The listing builds one solid part. Answer for the finished solid, in the listing's coordinates (mm). Give positions to 0.01 mm unless a question says otherwise; leave off trailing zeros. Loops run counter-clockwise (first coordinate to the right, second up) from the corner with the lowest first, then second, coordinate; pieces in that order, holes last. Notation, with made-up numbers: (76.5, -12.5) - (105.5, -12.5) arc R24 ccw to (105.5, 5.5) - close; hole circle Ø10 at (64, 1.25). An arc over 180 degrees is marked (long way). Write each question's results on one line, items separated by ' | '.
from build123d import *

# Parameters (mm, degrees)
F0_W     = 45
F0_H     = 60
F1_DEPTH = 3


with BuildPart() as f1:
    # F0 (on Top) → F1 (new body)
    with BuildSketch(Plane.XY):
        Rectangle(F0_W, F0_H)
        with BuildLine():
            ThreePointArc((-13.6944653346, -25.298272824), (-15.6944653346, -27.298272824), (-17.6944653346, -25.298272824))
            Line((-17.6944653346, -25.298272824), (-17.6944653346, -21.298272824))
            ThreePointArc((-17.6944653346, -21.298272824), (-17.1086788969, -19.8840592617), (-15.6944653346, -19.298272824))
            Line((-15.6944653346, -19.298272824), (-15.6944653346, 16.701727176))
            ThreePointArc((-15.6944653346, 16.701727176), (-17.1086788969, 17.2875136136), (-17.6944653346, 18.701727176))
            Line((-17.6944653346, 18.701727176), (-17.6944653346, 22.701727176))
            ThreePointArc((-17.6944653346, 22.701727176), (-15.6944653346, 24.701727176), (-13.6944653346, 22.701727176))
            Line((-13.6944653346, 22.701727176), (-13.6944653346, 20.701727176))
            Line((-13.6944653346, 20.701727176), (13.3055346654, 20.701727176))
            Line((13.3055346654, 20.701727176), (13.3055346654, 22.701727176))
            ThreePointArc((13.3055346654, 22.701727176), (15.3055346654, 24.701727176), (17.3055346654, 22.701727176))
            Line((17.3055346654, 22.701727176), (17.3055346654, 18.701727176))
            ThreePointArc((17.3055346654, 18.701727176), (16.7197482278, 17.2875136136), (15.3055346654, 16.701727176))
            Line((15.3055346654, 16.701727176), (15.3055346654, -19.298272824))
            ThreePointArc((15.3055346654, -19.298272824), (16.7197482278, -19.8840592617), (17.3055346654, -21.298272824))
            Line((17.3055346654, -21.298272824), (17.3055346654, -25.298272824))
            ThreePointArc((17.3055346654, -25.298272824), (15.3055346654, -27.298272824), (13.3055346654, -25.298272824))
            Line((13.3055346654, -25.298272824), (13.3055346654, -23.298272824))
            Line((13.3055346654, -23.298272824), (-13.6944653346, -23.298272824))
            Line((-13.6944653346, -23.298272824), (-13.6944653346, -25.298272824))
        make_face(mode=Mode.SUBTRACT)
        with BuildLine():
            Line((-13.6944653346, -21.298272824), (-13.6944653346, -23.298272824))
            Line((-13.6944653346, -23.298272824), (13.3055346654, -23.298272824))
            Line((13.3055346654, -23.298272824), (13.3055346654, -21.298272824))
            ThreePointArc((13.3055346654, -21.298272824), (13.8913211031, -19.8840592617), (15.3055346654, -19.298272824))
            Line((15.3055346654, -19.298272824), (15.3055346654, 16.701727176))
            ThreePointArc((15.3055346654, 16.701727176), (13.8913211031, 17.2875136136), (13.3055346654, 18.701727176))
            Line((13.3055346654, 18.701727176), (13.3055346654, 20.701727176))
            Line((13.3055346654, 20.701727176), (-13.6944653346, 20.701727176))
            Line((-13.6944653346, 20.701727176), (-13.6944653346, 18.701727176))
            ThreePointArc((-13.6944653346, 18.701727176), (-14.2802517722, 17.2875136136), (-15.6944653346, 16.701727176))
            Line((-15.6944653346, 16.701727176), (-15.6944653346, -19.298272824))
            ThreePointArc((-15.6944653346, -19.298272824), (-14.2802517722, -19.8840592617), (-13.6944653346, -21.298272824))
        make_face()
    extrude(amount=F1_DEPTH)


solid = f1.part
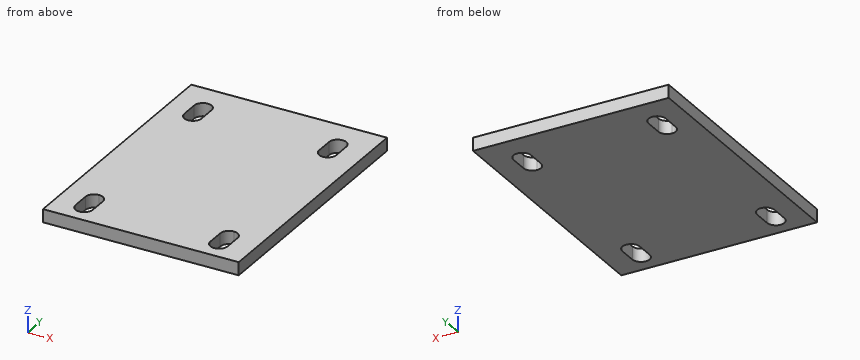
Item 1: Find the intervals of material crossed by line 1 along X through (y, z) = (20, 1); line 2 along X through (y, z) = (-19.5, 1.85); line 3 along Y through (x, z) = (-16, 0.95), in increasing order. Write a range as [from, to].
Values found:
line 1: x = [-22.5, -17.69], [-13.69, 13.31], [17.31, 22.5] | line 2: x = [-22.5, -16.57], [-14.82, 14.43], [16.18, 22.5] | line 3: y = [-30, -27.27], [-19.32, 16.73], [24.68, 30]
Item 2: A cutting plane is placed at C-C, the plane z = 1.55. Determine the outline of the cut face in (x, y).
Values found:
outline: (-22.5, -30) - (22.5, -30) - (22.5, 30) - (-22.5, 30) - close; hole (-17.69, -25.3) arc R2 ccw to (-13.69, -25.3) - (-13.69, -21.3) arc R2 ccw to (-17.69, -21.3) - close; hole (-17.69, 18.7) arc R2 ccw to (-13.69, 18.7) - (-13.69, 22.7) arc R2 ccw to (-17.69, 22.7) - close; hole (13.31, -25.3) arc R2 ccw to (17.31, -25.3) - (17.31, -21.3) arc R2 ccw to (13.31, -21.3) - close; hole (13.31, 18.7) arc R2 ccw to (17.31, 18.7) - (17.31, 22.7) arc R2 ccw to (13.31, 22.7) - close
Item 3: A cutting plane is placed at B-B, the plane x = 16.5. Determine the outline of the cut face in (y, z).
Values found:
outline: (-30, 0) - (-26.9, 0) - (-26.9, 3) - (-30, 3) - close; (-19.69, 0) - (17.1, 0) - (17.1, 3) - (-19.69, 3) - close; (24.31, 0) - (30, 0) - (30, 3) - (24.31, 3) - close
Item 4: A cutting plane is placed at A-A, the plane y = 21.5. Determine the outline of the cut face in (x, z).
Values found:
outline: (-22.5, 0) - (-17.69, 0) - (-17.69, 3) - (-22.5, 3) - close; (-13.69, 0) - (13.31, 0) - (13.31, 3) - (-13.69, 3) - close; (17.31, 0) - (22.5, 0) - (22.5, 3) - (17.31, 3) - close
